Check sheet for the modelled part. Datum: model origin and axes. Units: mm. A direction names the side the tool comes from. Give positions to 0.01 mm unless a question says otherwise; leave off trailing zeros. Loops run counter-clockwise (first coordinate to the right, second up) from the corner with the lowest first, then second, coordinate; pieces in that order, holes last. Notation, with made-up numbers: (82.5, 44.5) -> (124.5, 44.5) arc R17 cw to (124.5, 53.5) -> close; hole circle Ø6 at (85.5, 12). An arc over 180 degrees is marked (long way). Write each question's results on one line, items separated by ' | '. Start each with the question number.
1. Cross-section at A-A on z = 52.5. Count the separate pieces of the cut face and the enclosed holes in it, and give its area (3 significant figures).
2. Cross-section at D-D on z = 35. Record the boundary of the cut face in (x, y), and give its area (3 significant figures).
3. Cross-section at B-B on x = 30. Record the boundary of the cut face in (y, z), and give its area (3 significant figures).
4. Material ranges on L1, parallel to Z at x = 30, y = -0.45; L2, parallel to X at y = -4.5, z = 73.5; L3, parallel to X at y = -5.25, z = 55.5, recorded low to high. Write a range as from..to.
5. Gauge pin test, flat ends, axial feed: pin 1 Ø0.8 at (x, z) = (28, 87.5) entering from -Y; pin 2 Ø3 at (x, z) = (55.68, 85.68) entering from -Y; pin 3 Ø4 at (y, z) = (-8, 63.5) entering from +X. Record the tip position at first contact, or that the pin passes through.
6. Tool access check on faces 4 (the face through (57.861, -1.014, 87.745)), 5 (the face through (48, -6, 57.5)), 6 (the face through (30, -1, 25)), 7 (the face through (46, -6, 36)). Record the directions out of +Z, -Z, +X, -X, +Y, -Y that give a thin tool (end or side, any length) a straight path to the whole face; none if there is none.
7. Mould release check, pull along Z, two halves, no side actions. Record for faces 1 (the face through (38, -4, 48)), 2 (the face through (10, -6, 54)), 3 (the face through (22, -4, 49)): +Z half, -Z half, draft (parallel to the pull), parting line (faces both ways), or undercut.
from build123d import *

# Parameters (mm, degrees)
F0_W      = 60
F0_H      = 90
F1_DEPTH  = 2
F2_R      = 7.5
F4_W      = 2
F4_H      = 15
F5_DEPTH  = 25
F6_W      = 20
F6_H      = 40
F6_W_2    = 18
F6_H_2    = 38
F7_DEPTH  = 5
F8_W      = 8
F8_H      = 1
F9_DEPTH  = 3
F10_W     = 12
F10_H     = 1
F11_DEPTH = 5
F12_R     = 1.25
F13_DEPTH = 25
F14_W     = 6
F14_H     = 30
F15_DEPTH = 25
F16_R     = 3.75
F17_DEPTH = 25
F18_R     = 1.5
F19_DEPTH = 25
F20_W     = 4
F20_H     = 25
F21_DEPTH = 8
F22_R     = 1.5
F23_DEPTH = 25
F24_W     = 4
F24_H     = 10
F25_DEPTH = 8


with BuildPart() as f1:
    # F0 (on Front) → F1 (new body)
    with BuildSketch(Plane.XZ):
        with Locations((30, 45)):
            Rectangle(F0_W, F0_H)
    extrude(amount=F1_DEPTH)

    # F2
    f2_edges = [f1.edges().sort_by_distance(p)[0] for p in [
        (0, -1, 90),
        (60, -1, 90),
        (60, -1, 0),
        (0, -1, 0),
    ]]
    fillet(f2_edges, radius=F2_R)

    # F4 (on face) → F5 (cut)
    with BuildSketch(Plane.XZ.offset(2)):
        with Locations((19, 15)):
            Rectangle(F4_W, F4_H)
        with Locations((41, 15)):
            Rectangle(F4_W, F4_H)
    extrude(amount=-F5_DEPTH, mode=Mode.SUBTRACT)

    # F6 (on face) → F7 (join)
    with BuildSketch(Plane.XZ.offset(2)):
        with Locations((30, 68)):
            Rectangle(F6_W, F6_H)
        with Locations((30, 68)):
            Rectangle(F6_W_2, F6_H_2, mode=Mode.SUBTRACT)
    extrude(amount=F7_DEPTH)

    # F8 (on face) → F9 (cut)
    with BuildSketch(Plane.XZ.offset(7)):
        with Locations((30, 87.5)):
            Rectangle(F8_W, F8_H)
    extrude(amount=-F9_DEPTH, mode=Mode.SUBTRACT)

    # F10 (on face) → F11 (cut)
    with BuildSketch(Plane.XZ.offset(7)):
        with Locations((30, 48.5)):
            Rectangle(F10_W, F10_H)
    extrude(amount=-F11_DEPTH, mode=Mode.SUBTRACT)

    # F12 (on face) → F13 (cut)
    with BuildSketch(Plane.XZ.offset(2)):
        with Locations((7.146447, 82.853553)):
            Circle(F12_R)
        with Locations((52.853553, 82.853553)):
            Circle(F12_R)
        with Locations((55.681981, 4.318019)):
            Circle(F12_R)
        with Locations((4.318019, 4.318019)):
            Circle(F12_R)
        with Locations((7.146447, 7.146447)):
            Circle(F12_R)
        with Locations((52.853553, 7.146447)):
            Circle(F12_R)
        with Locations((55.681981, 85.681981)):
            Circle(F12_R)
        with Locations((4.318019, 85.681981)):
            Circle(F12_R)
    extrude(amount=-F13_DEPTH, mode=Mode.SUBTRACT)

    # F14 (on face) → F15 (cut)
    with BuildSketch(Plane.XZ.offset(2)):
        with Locations((30, 40)):
            Rectangle(F14_W, F14_H)
    extrude(amount=-F15_DEPTH, mode=Mode.SUBTRACT)

    # F16 (on face) → F17 (cut)
    with BuildSketch(Plane.XZ.offset(2)):
        with Locations((30, 80)):
            Circle(F16_R)
    extrude(amount=-F17_DEPTH, mode=Mode.SUBTRACT)

    # F18 (on face) → F19 (cut)
    with BuildSketch(Plane.XZ.offset(2)):
        with Locations((5, 17.5)):
            Circle(F18_R)
        with Locations((5, 72.5)):
            Circle(F18_R)
        with Locations((55, 72.5)):
            Circle(F18_R)
        with Locations((55, 17.5)):
            Circle(F18_R)
    extrude(amount=-F19_DEPTH, mode=Mode.SUBTRACT)

    # F20 (on face) → F21 (join)
    with BuildSketch(Plane.XZ.offset(2)):
        with Locations((12, 45)):
            Rectangle(F20_W, F20_H)
        with Locations((48, 45)):
            Rectangle(F20_W, F20_H)
    extrude(amount=F21_DEPTH)

    # F22 (on face) → F23 (cut)
    with BuildSketch(Plane.XZ.offset(2)):
        with Locations((5, 52.5)):
            Circle(F22_R)
        with Locations((5, 37.5)):
            Circle(F22_R)
        with Locations((55, 52.5)):
            Circle(F22_R)
        with Locations((55, 37.5)):
            Circle(F22_R)
    extrude(amount=-F23_DEPTH, mode=Mode.SUBTRACT)

    # F24 (on face) → F25 (cut)
    with BuildSketch(Plane.XZ.offset(10)):
        with Locations((12, 45)):
            Rectangle(F24_W, F24_H)
        with Locations((48, 45)):
            Rectangle(F24_W, F24_H)
    extrude(amount=-F25_DEPTH, mode=Mode.SUBTRACT)


solid = f1.part
Geometry says:
1) separate pieces: 4 | enclosed holes: 0 | area: 170 mm^2
2) outline: (0, -2) -> (10, -2) -> (10, -10) -> (14, -10) -> (14, -2) -> (27, -2) -> (27, 0) -> (0, 0) -> close; (33, -2) -> (46, -2) -> (46, -10) -> (50, -10) -> (50, -2) -> (60, -2) -> (60, 0) -> (33, 0) -> close | area: 172 mm^2
3) outline: (-4, 87) -> (-2, 87) -> (-2, 83.75) -> (0, 83.75) -> (0, 90) -> (-2, 90) -> (-2, 88) -> (-4, 88) -> close; (-2, 0) -> (0, 0) -> (0, 25) -> (-2, 25) -> close; (-2, 55) -> (0, 55) -> (0, 76.25) -> (-2, 76.25) -> close | area: 107 mm^2
4) L1: 0..25, 55..76.25, 83.75..90 | L2: 20..21, 39..40 | L3: 10..14, 20..21, 39..40, 46..50
5) pin 1: y = -4 | pin 2: y = -2 | pin 3: x = 40
6) face 4: +Z, +X, +Y, -Y | face 5: +Z, +X, -Y | face 6: +Y, -Y | face 7: +Z, -Z, -Y
7) face 1: -Z half | face 2: draft | face 3: undercut
